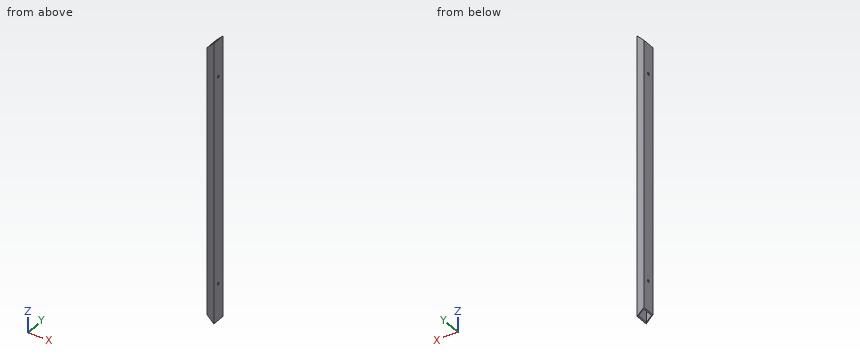
Autodesk Inventor part; units mm, degrees
ref_plane "YZ Plane" through (0, 0, 0) normal (1, 0, 0) x (0, 1, 0)
ref_plane "XZ Plane" through (0, 0, 0) normal (0, 1, 0) x (-1, 0, 0)
ref_plane "XY Plane" through (0, 0, 0) normal (0, 0, 1) x (1, 0, 0)
sketch "Sketch2" plane through (0, 0, 0) normal (0, 0, 1) x (1, 0, 0)
  line L0 (-4.1078, 5.9023) -> (21.2922, 5.9023)
  line L1 (21.2922, 5.9023) -> (21.2922, -44.8977)
  line L2 (21.2922, -44.8977) -> (-4.1078, -44.8977)
  line L3 (-4.1078, -44.8977) -> (-4.1078, 5.9023)
  line L4 (18.1934, 2.8035) -> (-1.009, 2.8035)
  line L5 (-1.009, 2.8035) -> (-1.009, -41.7989)
  line L6 (-1.009, -41.7989) -> (18.1934, -41.7989)
  line L7 (18.1934, -41.7989) -> (18.1934, 2.8035)
  point P0 (0, 0)
  dimension "d0" = 25.4
  dimension "d1" = 50.8
  dimension "d2" = 3.0988
extrude "Extrusion1" add sketch "Sketch2" along normal blind 1066.8
sketch "Sketch5" plane through (0, 0, 1066.8) normal (0, 0, 1) x (1, 0, 0)
  point P0 (0, 0)
sketch "Sketch6" plane through (-4.1078, 5.9023, 0) normal (0, 1, 0) x (1, 0, 0)
  line L0 (25.4, 0) -> (-1.2066, -26.6066)
  line L1 (0, 0) -> (0, -1066.8)
  line L2 (0, -25.4) -> (0, 0)
  line L3 (0, 0) -> (25.4, 0)
  line L4 (0, -1066.8) -> (25.4, -1066.8)
  line L5 (25.4, -1066.8) -> (-7.0638, -1034.3362)
  line L6 (25.4, -1066.8) -> (71.3108, -1066.8) construction
  line L7 (0, -1041.4) -> (0, -1066.8)
  line L8 (0, -1066.8) -> (25.4, -1066.8)
  point P0 (4.1078, 0)
  dimension "d11" = 135
extrude "Extrusion2" cut sketch "Sketch6" against normal blind 1066.8 contours L0 L1 L3
extrude "Extrusion3" cut sketch "Sketch6" against normal blind 1066.8 contours L5 L4 L1
sketch "Sketch7" plane through (21.2922, -44.8977, 0) normal (1, 0, 0) x (0, 0, -1)
  line L0 (0, 0) -> (-1066.8, 0)
  line L1 (0, 50.4825) -> (-139.7, 50.4825)
  line L2 (-139.7, 50.4825) -> (-139.7, 0)
  line L3 (-139.7, 0) -> (0, 0)
  line L4 (0, 0) -> (0, 50.4825)
  line L5 (-1066.8, 50.4825) -> (-927.1, 50.4825)
  line L6 (-927.1, 50.4825) -> (-927.1, -0.3175)
  line L7 (-927.1, -0.3175) -> (-1066.8, -0.3175)
  line L8 (-1066.8, -0.3175) -> (-1066.8, 50.4825)
  point P0 (0, 44.8977)
  point P1 (-139.7, 25.2412)
  point P2 (-927.1, 25.0825)
  dimension "d12" = 139.7
  dimension "d13" = 139.7
  dimension "d14" = 50.8
hole "Hole1" at (21.2922, -19.8152, 927.1) at (21.2922, -19.6564, 139.7) direction (-1, 0, 0) diameter 9.525 end through all
properties part number "42in 2x1 boxbeam"
Geometry check sheet. Reference: the model listing, model coordinates, mm. Give positions to 0.01 mm unless a question says otherwise; leave off trailing zeros. Write each loop counter-clockwise with the first axis right and the second up, starting at its lowest first coordinate (ties: lowest second). Pieces come first, ordered by that corner, then holes. Notation, with made-up numbers: (3, -20) - (38, -20) arc R28 cw to (38, 7) - close; hole circle Ø4 at (-14, 14.25). An arc over 180 degrees is marked (long way). Use a Markdown table: item, result.
Q1. Thickness scan on L1, parallel to Y at x = 17.25, z = 590.5; L2, parallel to Y at x = 19.45, z = 927.1; L3, parallel to Z at x = -1.25, y = -22. Record the ranges inside material, lowest first. Write a range as [from, to].
Computed:
| item | result |
|---|---|
| L1 | y = [-44.9, -41.8], [2.8, 5.9] |
| L2 | y = [-44.9, -24.58], [-15.05, 5.9] |
| L3 | z = [22.54, 135.55], [143.85, 922.87], [931.33, 1044.26] |
Q2. Section check A-A, the plane z = 532. Enter the section's corners in (x, y), then the cut area to 3 significant figures.
Computed:
| item | result |
|---|---|
| outline | (-4.11, -44.9) - (21.29, -44.9) - (21.29, 5.9) - (-4.11, 5.9) - close; hole (-1.01, -41.8) - (18.19, -41.8) - (18.19, 2.8) - (-1.01, 2.8) - close |
| area | 434 mm² |
Q3. Section check B-B, the plane x = 12.25. Enter the section's corners in (y, z), then the cut area to 3 significant figures.
Computed:
| item | result |
|---|---|
| outline | (-44.9, 9.04) - (-41.8, 9.04) - (-41.8, 1057.76) - (-44.9, 1057.76) - close; (2.8, 9.04) - (5.9, 9.04) - (5.9, 1057.76) - (2.8, 1057.76) - close |
| area | 6,500 mm² |
Q4. Go/stop test with a flat-tipped pin: P1, Ø6, axis at x = 14.5, y = -13, coming from the -Z side. Record where the tip stops, or that it passes through.
Computed:
| item | result |
|---|---|
| P1 | passes through |
